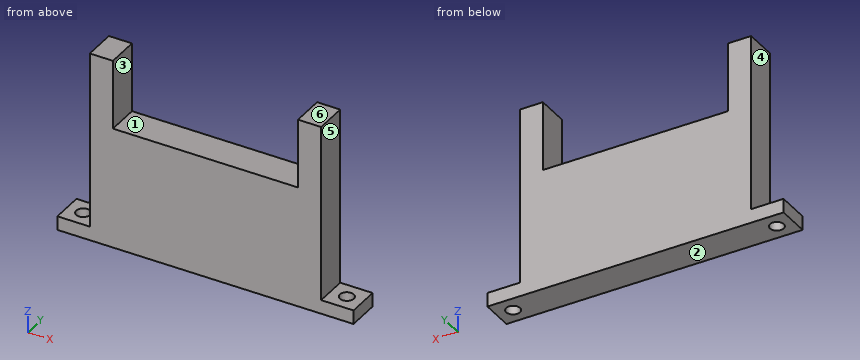
from build123d import *

# Parameters (mm, degrees)
SKETCH_1_W          = 64
SKETCH_1_H          = 7
EXTRUDE_3_DEPTH     = 3
SKETCH_3_W          = 50
SKETCH_3_H          = 7
EXTRUDE_4_DEPTH     = 23.3
SKETCH_4_W          = 5
SKETCH_4_H          = 7
EXTRUDE_5_DEPTH     = 15
SKETCH_5_W          = 5
SKETCH_5_H          = 7
EXTRUDE_6_DEPTH     = 15
SKETCH_6_R          = 1.5
CUT_EXTRUDE_1_DEPTH = 3
SKETCH_7_R          = 1.5
CUT_EXTRUDE_2_DEPTH = 3


with BuildPart() as part:
    # Эскиз1 → Бобышка-Вытянуть3 (new body)
    with BuildSketch(Plane.XY):
        Rectangle(SKETCH_1_W, SKETCH_1_H)
    extrude(amount=EXTRUDE_3_DEPTH)

    # Эскиз3 → Бобышка-Вытянуть4 (add)
    with BuildSketch(Plane.XY.offset(3)):
        Rectangle(SKETCH_3_W, SKETCH_3_H)
    extrude(amount=EXTRUDE_4_DEPTH)

    # Эскиз4 → Бобышка-Вытянуть5 (add)
    with BuildSketch(Plane.XY.offset(26.3)):
        with Locations((-22.5, 0)):
            Rectangle(SKETCH_4_W, SKETCH_4_H)
    extrude(amount=EXTRUDE_5_DEPTH)

    # Эскиз5 → Бобышка-Вытянуть6 (add)
    with BuildSketch(Plane.XY.offset(26.3)):
        with Locations((22.5, 0)):
            Rectangle(SKETCH_5_W, SKETCH_5_H)
    extrude(amount=EXTRUDE_6_DEPTH)

    # Эскиз6 → Вырез-Вытянуть1 (cut)
    with BuildSketch(Plane.XY.offset(3)):
        with Locations((-28.5, 0)):
            Circle(SKETCH_6_R)
    extrude(amount=-CUT_EXTRUDE_1_DEPTH, mode=Mode.SUBTRACT)

    # Эскиз7 → Вырез-Вытянуть2 (cut)
    with BuildSketch(Plane.XY.offset(3)):
        with Locations((28.5, 0)):
            Circle(SKETCH_7_R)
    extrude(amount=-CUT_EXTRUDE_2_DEPTH, mode=Mode.SUBTRACT)


solid = part.part
Input: part model. Units: mm. Frame: model coordinates. Face numbers are marked on the shaded views. A direction names the side the tool comes from. Coordinates: 2 decimals unless noted, no trailing zeros. Loops run counter-clockwise (first coordinate to the right, second up) from the corner with the lowest first, then second, coordinate; pieces in that order, holes last. Notation, with made-up numbers: (-17.75, -1) -> (21.25, -1) arc R21 ccw to (21.25, 4) -> close; hole circle Ø3 at (-19, -5.5). An arc over 180 degrees is marked (long way). Write each question's results on one line, items separated by ' | '. Start each with the question number.
Q1. Ray query, line 1 (X direction, y = 2.75, z = 33); line 2 (Y direction, x = -28.5, z = 1.8); line 3 (X direction, y = -0.5, z = 21). Return the intervals inside material, ascending. Write a range as from..to.
Q2. Pull-direction query (X, two-part tool) for the marked faces 3, 4, 5 and 6; classes: released by +X, released by -X, zero draft, split by the parting line, or undercut.
Q3. Section C-C, the plane y = 0. Return the cut outline in (x, z), plus the area to 3 significant figures.
Q4. Reachability of the marked faces 1 and 2 from +Z, -Z, +X, -X, +Y, -Y: full face, straight path, thin tool, end or side. Return the list, or none.
Q5. Section A-A, the plane z = 27.5. Return the cut outline in (x, y).
Q6. Pin query (flat end, axial travel): pin 1 (1 mm diameter, centred on x = 6.5, y = -0.5, fed in from +Z); pin 2 (2 mm diameter, centred on y = 2, z = 13, fed in from -X); pin 3 (2.5 mm diameter, centred on x = -28.5, y = 0, fed in from +Z); pin 4 (3.5 mm diameter, centred on x = 29, y = 1, fed in from +Z). Return the tip coordinate at first contact, or that it passes through.
Q7. Section B-B, the plane x = -28.5. Return the cut outline in (y, z), plus the area to 3 significant figures.
Q8. Section D-D, the plane x = 3.5. Return the cut outline in (y, z).
Found:
1) line 1: -25..-20, 20..25 | line 2: -3.5..-1.5, 1.5..3.5 | line 3: -25..25
2) face 3: undercut | face 4: released by -X | face 5: released by +X | face 6: zero draft
3) outline: (-32, 0) -> (-30, 0) -> (-30, 3) -> (-32, 3) -> close; (-27, 0) -> (27, 0) -> (27, 3) -> (25, 3) -> (25, 41.3) -> (20, 41.3) -> (20, 26.3) -> (-20, 26.3) -> (-20, 41.3) -> (-25, 41.3) -> (-25, 3) -> (-27, 3) -> close; (30, 0) -> (32, 0) -> (32, 3) -> (30, 3) -> close | area: 1,490 mm2
4) face 1: +Z, +Y, -Y | face 2: -Z, +X, -X, +Y, -Y
5) outline: (-25, -3.5) -> (-20, -3.5) -> (-20, 3.5) -> (-25, 3.5) -> close; (20, -3.5) -> (25, -3.5) -> (25, 3.5) -> (20, 3.5) -> close
6) pin 1: z = 26.3 | pin 2: x = -25 | pin 3: through | pin 4: z = 3
7) outline: (-3.5, 0) -> (-1.5, 0) -> (-1.5, 3) -> (-3.5, 3) -> close; (1.5, 0) -> (3.5, 0) -> (3.5, 3) -> (1.5, 3) -> close | area: 12.0 mm2
8) outline: (-3.5, 0) -> (3.5, 0) -> (3.5, 26.3) -> (-3.5, 26.3) -> close
